Model file for the job. Use its own axes, mm. Face numbers are marked on the shaded views. A direction names the side the tool comes from. Round coordinates to 2 decimals unless told otherwise and drop trailing zeros. Write each loop counter-clockwise with the first axis right and the second up, starting at its lowest first coordinate (ties: lowest second). Pieces come first, ordered by that corner, then holes.
```python
from build123d import *

# Parameters (mm, degrees)
SKETCH1_W           = 8
SKETCH1_H           = 8
BOSS_EXTRUDE1_DEPTH = 8
SKETCH2_W           = 3.95
SKETCH2_H           = 3.95
BOSS_EXTRUDE2_DEPTH = 2.4
SKETCH3_W           = 2.95
SKETCH3_H           = 1.95
BOSS_EXTRUDE3_DEPTH = 3
SKETCH4_R           = 0.28
BOSS_EXTRUDE4_DEPTH = 3.75


with BuildPart() as part:
    # Sketch1 → Boss-Extrude1 (new body)
    with BuildSketch(Plane(origin=(0, 0, 0), x_dir=(1, 0, 0), z_dir=(0, 1, 0))):
        Rectangle(SKETCH1_W, SKETCH1_H)
    extrude(amount=BOSS_EXTRUDE1_DEPTH)

    # Sketch2 → Boss-Extrude2 (add)
    with BuildSketch(Plane(origin=(0, 8, 0), x_dir=(1, 0, 0), z_dir=(0, 1, 0))):
        Rectangle(SKETCH2_W, SKETCH2_H)
    extrude(amount=BOSS_EXTRUDE2_DEPTH)

    # Sketch3 → Boss-Extrude3 (add)
    with BuildSketch(Plane(origin=(0, 10.4, 0), x_dir=(1, 0, 0), z_dir=(0, 1, 0))):
        Rectangle(SKETCH3_W, SKETCH3_H)
    extrude(amount=BOSS_EXTRUDE3_DEPTH)

    # Sketch4 → Boss-Extrude4 (add)
    with BuildSketch(Plane.XZ):
        with Locations(Location((2.54, 2.54, 0), (0, 0, 270))):
            Circle(SKETCH4_R)
        with Locations(Location((2.54, 0, 0), (0, 0, 270))):
            Circle(SKETCH4_R)
        with Locations(Location((2.54, -2.54, 0), (0, 0, 270))):
            Circle(SKETCH4_R)
        with Locations(Location((-2.54, -2.54, 0), (0, 0, 270))):
            Circle(SKETCH4_R)
        with Locations(Location((-2.54, 0, 0), (0, 0, 270))):
            Circle(SKETCH4_R)
        with Locations(Location((-2.54, 2.54, 0), (0, 0, 270))):
            Circle(SKETCH4_R)
    extrude(amount=BOSS_EXTRUDE4_DEPTH)


solid = part.part
```
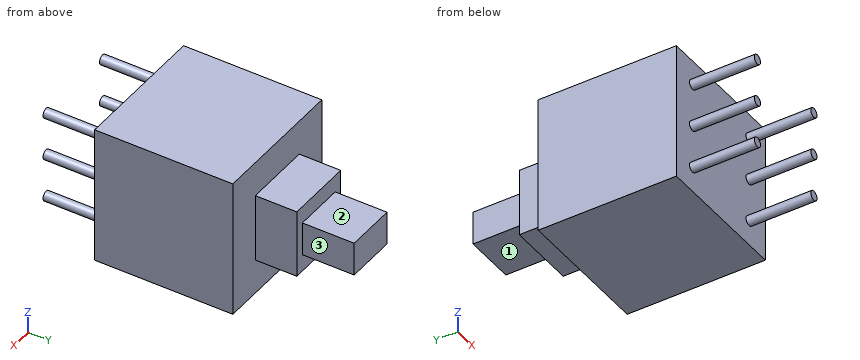
1) Cut at D-D on x = 1. List the corners of the cut face in (y, z) (3 decimals), and give its area (3 significant figures).
2) Cut at A-A on y = -1. List the corners of the cut face in (x, z).
3) Wall check: probe 1 along X at (y, z) = (-0.75, 2.5); probe 2 along Y at (x, z) = (-1, -3.25); probe 3 along Y at (x, z) = (-0.75, 0.25). Give the ranges that are in metal, low to high.
4) Cut at C-C on x = 2.54. List the corners of the cut face in (y, z).
5) Flat gauge pins, fed straight in: pin 1 Ø1.5 at (x, y) = (0, 11.5) entering from +Z (3 decimals); pin 2 Ø0.9 at (x, y) = (-0.5, 12.5) entering from -Z (3 decimals); pin 3 Ø1.5 at (x, z) = (1.5, -1) entering from -Y. Where does each tip first touch, or does it go through?
6) Cut at B-B on z = -2.54. List the corners of the cut face in (x, y).
7) Which spindle directions (+Z, -Z, +X, -X, +Y, -Y) get a long thin tool onto all of the face, cutting with end or side? Do the marked faces 1, 2 and 3. Say none if no direction does.
Result sheet:
1. outline: (0, -4) - (8, -4) - (8, -1.975) - (10.4, -1.975) - (10.4, -0.975) - (13.4, -0.975) - (13.4, 0.975) - (10.4, 0.975) - (10.4, 1.975) - (8, 1.975) - (8, 4) - (0, 4) - close
1. area: 79.3 mm2
2. outline: circle Ø0.56 at (-2.54, -2.54); circle Ø0.56 at (-2.54, 0); circle Ø0.56 at (-2.54, 2.54); circle Ø0.56 at (2.54, -2.54); circle Ø0.56 at (2.54, 0); circle Ø0.56 at (2.54, 2.54)
3. probe 1: x = -2.82 to -2.26, 2.26 to 2.82
3. probe 2: y = 0 to 8
3. probe 3: y = 0 to 13.4
4. outline: (-3.75, -2.82) - (0, -2.82) - (0, -4) - (8, -4) - (8, 4) - (0, 4) - (0, 2.82) - (-3.75, 2.82) - (-3.75, 2.26) - (0, 2.26) - (0, 0.28) - (-3.75, 0.28) - (-3.75, -0.28) - (0, -0.28) - (0, -2.26) - (-3.75, -2.26) - close
5. pin 1: stops at z = 0.975
5. pin 2: stops at z = -0.975
5. pin 3: stops at y = 0
6. outline: (-4, 0) - (-2.82, 0) - (-2.82, -3.75) - (-2.26, -3.75) - (-2.26, 0) - (2.26, 0) - (2.26, -3.75) - (2.82, -3.75) - (2.82, 0) - (4, 0) - (4, 8) - (-4, 8) - close
7. face 1: -Z, +X, -X, +Y
7. face 2: +Z, +X, -X, +Y
7. face 3: +Z, -Z, +X, +Y
